```python
from build123d import *
from build123d.topology import SkipClean

# Parameters (mm, degrees)
DODANIE_WYCI_GNI_CIE1_DEPTH = 2
SZKIC_START                 = -28.065385
SZKIC_ZGI_CIA1_DEPTH        = 54
SZKIC_ZGI_CIA1_2_DEPTH      = 15.5
SZKIC_START_2               = 10.434615
SZKIC_ZGI_CIA1_3_DEPTH      = 15.5
SZKIC_START_3               = -56.031828
SZKIC_ZGI_CIA1_4_DEPTH      = 2.423909
SZKIC_START_4               = -12.565385
SZKIC_ZGI_CIA1_5_DEPTH      = 23
SZKIC_ZGI_CIA1_6_DEPTH      = 23
SZKIC_ZGI_CIA2_DEPTH        = 54
SZKIC_ZGI_CIA2_2_DEPTH      = 54
SZKIC_START_5               = 49.968172
SZKIC_ZGI_CIA2_3_DEPTH      = 2
SZKIC9_W                    = 87
SZKIC9_H                    = 28
SZKIC9_W_2                  = 15
SZKIC9_H_2                  = 7
WYTNIJ_WYCI_GNI_CIE1_DEPTH  = 66.825561
SZKIC10_R                   = 1.5
WYTNIJ_WYCI_GNI_CIE2_DEPTH  = 114.762973
ZAOKR_GLENIE2_R             = 1
ZAOKR_GLENIE3_R             = 1


with BuildPart() as part:
    # Szkic1 → Dodanie-wyciągnięcie1 (new body)
    with BuildSketch(Plane.XY):
        with BuildLine():
            Line((-75.531828, 25.934615), (71.468172, 25.934615))
            Line((71.468172, 25.934615), (71.468172, 10.434615))
            ThreePointArc((71.468172, 10.434615), (59.968172, -1.065385), (71.468172, -12.565385))
            Line((71.468172, -12.565385), (71.468172, -28.065385))
            Line((71.468172, -28.065385), (-75.531828, -28.065385))
            Line((-75.531828, -28.065385), (-75.531828, -12.565385))
            ThreePointArc((-75.531828, -12.565385), (-64.031828, -1.065385), (-75.531828, 10.434615))
            Line((-75.531828, 10.434615), (-75.531828, 25.934615))
        make_face()
    extrude(amount=DODANIE_WYCI_GNI_CIE1_DEPTH)

    # Szkic zgięcia1: read off the stored shape, not the designer's step
    # Szkic zgięcia1 outline → Szkic zgięcia1 (cut)
    with BuildSketch(Plane(origin=(0, 0, 0), x_dir=(1, 0, 0), z_dir=(0, 1, 0)).offset(SZKIC_START)):
        with BuildLine():
            Line((-75.531828, -2), (-55.981318, -2))
            ThreePointArc((-55.981318, -2), (-55.112967, -0.563508), (-53.531828, 0))
            Line((-53.531828, 0), (-75.531828, 0))
            Line((-75.531828, 0), (-75.531828, -2))
        make_face()
    extrude(amount=SZKIC_ZGI_CIA1_DEPTH, mode=Mode.SUBTRACT)

    # Szkic zgi_cia1 2 outline → Szkic zgi_cia1 2 (add)
    with BuildSketch(Plane(origin=(0, 0, 0), x_dir=(1, 0, 0), z_dir=(0, 1, 0)).offset(SZKIC_START)):
        with BuildLine():
            ThreePointArc((-55.981318, -2), (-56.019168, -2.248728), (-56.031828, -2.5))
            Line((-56.031828, -2.5), (-56.031828, -22.143806))
            Line((-56.031828, -22.143806), (-54.031828, -22.143806))
            Line((-54.031828, -22.143806), (-54.031828, -2.5))
            ThreePointArc((-54.031828, -2.5), (-53.885381, -2.146447), (-53.531828, -2))
            Line((-53.531828, -2), (-55.981318, -2))
        make_face()
    extrude(amount=SZKIC_ZGI_CIA1_2_DEPTH)

    # Szkic zgi_cia1 3 outline → Szkic zgi_cia1 3 (add)
    with BuildSketch(Plane(origin=(0, 0, 0), x_dir=(1, 0, 0), z_dir=(0, 1, 0)).offset(SZKIC_START_2)):
        with BuildLine():
            ThreePointArc((-55.981318, -2), (-56.019168, -2.248728), (-56.031828, -2.5))
            Line((-56.031828, -2.5), (-56.031828, -22.143806))
            Line((-56.031828, -22.143806), (-54.031828, -22.143806))
            Line((-54.031828, -22.143806), (-54.031828, -2.5))
            ThreePointArc((-54.031828, -2.5), (-53.885381, -2.146447), (-53.531828, -2))
            Line((-53.531828, -2), (-55.981318, -2))
        make_face()
    extrude(amount=SZKIC_ZGI_CIA1_3_DEPTH)

    # Szkic zgi_cia1 4 outline → Szkic zgi_cia1 4 (add)
    with BuildSketch(Plane.YZ.offset(SZKIC_START_3)):
        with BuildLine():
            Line((10.434615, 2), (10.434615, 22.143806))
            ThreePointArc((10.434615, 22.143806), (-1.065385, 10.643806), (-12.565385, 22.143806))
            Line((-12.565385, 22.143806), (-12.565385, 2))
            Line((-12.565385, 2), (10.434615, 2))
        make_face()
    extrude(amount=SZKIC_ZGI_CIA1_4_DEPTH)

    # Szkic zgi_cia1 5 outline → Szkic zgi_cia1 5 (cut)
    with SkipClean():  # the faces are left unmerged after this step: merging them gives an invalid solid
        with BuildSketch(Plane(origin=(0, 0, 0), x_dir=(1, 0, 0), z_dir=(0, 1, 0)).offset(SZKIC_START_4)):
            with BuildLine():
                ThreePointArc((-53.607919, -2.005824), (-53.911331, -2.174459), (-54.031828, -2.5))
                Line((-54.031828, -2.5), (-54.031828, -24))
                Line((-54.031828, -24), (-53.607919, -24))
                Line((-53.607919, -24), (-53.607919, -2.005824))
            make_face()
            with BuildLine():
                Line((-58, -24), (-56.031828, -24))
                Line((-56.031828, -24), (-56.031828, -2.5))
                ThreePointArc((-56.031828, -2.5), (-56.019168, -2.248728), (-55.981318, -2))
                Line((-55.981318, -2), (-58, -2))
                Line((-58, -2), (-58, -24))
            make_face()
        extrude(amount=SZKIC_ZGI_CIA1_5_DEPTH, mode=Mode.SUBTRACT)

    # Szkic zgi_cia1 6 outline → Szkic zgi_cia1 6 (add)
    with SkipClean():  # the faces are left unmerged after this step: merging them gives an invalid solid
        with BuildSketch(Plane(origin=(0, 0, 0), x_dir=(1, 0, 0), z_dir=(0, 1, 0)).offset(SZKIC_START_4)):
            with BuildLine():
                Line((-53.607919, -2), (-53.607919, -2.005824))
                ThreePointArc((-53.607919, -2.005824), (-53.569985, -2.001458), (-53.531828, -2))
                Line((-53.531828, -2), (-53.607919, -2))
            make_face()
        extrude(amount=SZKIC_ZGI_CIA1_6_DEPTH)

    # Szkic zgięcia2: read off the stored shape, not the designer's step
    # Szkic zgięcia2 outline → Szkic zgięcia2 (cut)
    with SkipClean():  # the faces are left unmerged after this step: merging them gives an invalid solid
        with BuildSketch(Plane(origin=(0, 0, 0), x_dir=(1, 0, 0), z_dir=(0, 1, 0)).offset(SZKIC_START)):
            with BuildLine():
                ThreePointArc((49.468172, 0), (51.049311, -0.563508), (51.917662, -2))
                Line((51.917662, -2), (71.468172, -2))
                Line((71.468172, -2), (71.468172, 0))
                Line((71.468172, 0), (49.468172, 0))
            make_face()
        extrude(amount=SZKIC_ZGI_CIA2_DEPTH, mode=Mode.SUBTRACT)

    # Szkic zgi_cia2 2 outline → Szkic zgi_cia2 2 (add)
    with SkipClean():  # the faces are left unmerged after this step: merging them gives an invalid solid
        with BuildSketch(Plane(origin=(0, 0, 0), x_dir=(1, 0, 0), z_dir=(0, 1, 0)).offset(SZKIC_START)):
            with BuildLine():
                Line((49.968172, -22.143806), (51.968172, -22.143806))
                Line((51.968172, -22.143806), (51.968172, -2.5))
                ThreePointArc((51.968172, -2.5), (51.955512, -2.248728), (51.917662, -2))
                Line((51.917662, -2), (49.468172, -2))
                ThreePointArc((49.468172, -2), (49.821725, -2.146447), (49.968172, -2.5))
                Line((49.968172, -2.5), (49.968172, -22.143806))
            make_face()
        extrude(amount=SZKIC_ZGI_CIA2_2_DEPTH)

    # Szkic zgi_cia2 3 outline → Szkic zgi_cia2 3 (cut)
    with SkipClean():  # the faces are left unmerged after this step: merging them gives an invalid solid
        with BuildSketch(Plane.YZ.offset(SZKIC_START_5)):
            with BuildLine():
                Line((10.434615, 22.143806), (-12.565385, 22.143806))
                ThreePointArc((-12.565385, 22.143806), (-1.065385, 10.643806), (10.434615, 22.143806))
            make_face()
        extrude(amount=SZKIC_ZGI_CIA2_3_DEPTH, mode=Mode.SUBTRACT)

    # Szkic9 → Wytnij-wyciągnięcie1 (cut, through all)
    with SkipClean():  # the faces are left unmerged after this step: merging them gives an invalid solid
        with BuildSketch(Plane.XY.offset(2)):
            with Locations((-2.031828, -1.065385)):
                Rectangle(SZKIC9_W, SZKIC9_H)
            with Locations((35.468172, 22.434615)):
                Rectangle(SZKIC9_W_2, SZKIC9_H_2)
            with BuildLine():
                Line((-11.015655, 18.934615), (3.951999, 18.934615))
                ThreePointArc((3.951999, 18.934615), (4.951999, 17.934615), (3.951999, 16.934615))
                Line((3.951999, 16.934615), (-11.015655, 16.934615))
                ThreePointArc((-11.015655, 16.934615), (-12.015655, 17.934615), (-11.015655, 18.934615))
            make_face()
            with BuildLine():
                Line((-9.515655, -19.065385), (5.451999, -19.065385))
                ThreePointArc((5.451999, -19.065385), (6.451999, -20.065385), (5.451999, -21.065385))
                Line((5.451999, -21.065385), (-9.515655, -21.065385))
                ThreePointArc((-9.515655, -21.065385), (-10.515655, -20.065385), (-9.515655, -19.065385))
            make_face()
        extrude(amount=-WYTNIJ_WYCI_GNI_CIE1_DEPTH, mode=Mode.SUBTRACT)

    # Szkic10 → Wytnij-wyciągnięcie2 (cut, through all)
    with SkipClean():  # the faces are left unmerged after this step: merging them gives an invalid solid
        with BuildSketch(Plane.ZY.offset(56.031828)):
            with Locations((7.643806, 14.434615)):
                Circle(SZKIC10_R)
            with Locations((7.643806, -16.565385)):
                Circle(SZKIC10_R)
        extrude(amount=-WYTNIJ_WYCI_GNI_CIE2_DEPTH, mode=Mode.SUBTRACT)

    # Zaokrąglenie2
    zaokr_glenie2_edges = [part.edges().sort_by_distance(p)[0] for p in [
        (27.968172, 25.934615, 1),
        (42.968172, 25.934615, 1),
    ]]
    fillet(zaokr_glenie2_edges, radius=ZAOKR_GLENIE2_R)

    # Zaokrąglenie3
    zaokr_glenie3_edges = [part.edges().sort_by_distance(p)[0] for p in [
        (-45.531828, -15.065385, 1),
        (-45.531828, 12.934615, 1),
        (41.468172, 12.934615, 1),
        (41.468172, -15.065385, 1),
    ]]
    fillet(zaokr_glenie3_edges, radius=ZAOKR_GLENIE3_R)


solid = part.part
```
Geometry: final body of the model. Coordinates: model frame, mm. A direction names the side the tool comes from. Round coordinates to 2 decimals unless told otherwise and drop trailing zeros. Order: outer loops, then holes, each group sorted by start corner. A loop starts at its lowest first (then second) coordinate and runs counter-clockwise, first axis right, second up. Notation, with made-up numbers: M -21.75,15.25 L -12.75,15.25 A25 cw -12.75,52.25 Z; hole C 17,72 d8. An arc over 180 degrees is marked long. Use one line per item in the form item = value. Start each with the question number.
Q1. Cut plane B-B (z = 4.25). Return loops of the section in (x, y).
Q2. Pin query (flat end, axial travel): pin 1 Ø2 at (x, z) = (36.5, 0.5) entering from +Y; pin 2 Ø2 at (y, z) = (0.5, 1) entering from -X; pin 3 Ø2 at (y, z) = (21.5, 0.5) entering from +X. Return the tip coordinate at first contact, or that it passes through.
Q3. Cut plane A-A (y = 22.5). Return loops of the section in (x, z), and give its area (3 significant figures).
Q4. Material intervals for line 1 (X direction, y = 20, z = 16.75); line 2 (Z direction, x = -11, y = 21.5), sorted ascending. Write a range as [from, to].
Q5. Cut plane C-C (x = 7.5). Return loops of the section in (y, z).
Q6. Mould query, pull axis Z, two halves, no side actions, for faces 1 (the face through (-4, 18.935, 1)), 2 (the face through (-55, -20, 22.144)), 3 (the face through (-55.046, 15.922, 7.449)). Classes: +Z half, -Z half, draft (parallel to the pull), parting line (faces both ways), or undercut.
Q7. Cut plane D-D (z = 15.75). Return loops of the section in (x, y).
Q8. Access query for faces 4 (the face through (-1.3, -18.7, 2)), 5 (the face through (-55.13, -1.44, 0.58)), 6 (the face through (-3, -15.065, 1)). Directions: +Z, -Z, +X, -X, +Y, -Y. A direction counts if a zero-diameter tool reaches every point of the face in a straight line with its end or side. Return the directions, or none.
Geometry results:
q1.outline = M -56.03,-28.07 L -54.03,-28.07 L -54.03,25.93 L -56.03,25.93 Z; M 49.97,-28.07 L 51.97,-28.07 L 51.97,25.93 L 49.97,25.93 Z
q2.pin_1 = 18.93
q2.pin_2 = -55.98
q2.pin_3 = 51.76
q3.outline = M -56.03,2.5 A2.5 ccw -55.98,2 A2.5 ccw -53.53,0 L 27.97,0 L 27.97,2 L -53.53,2 A0.5 cw -54.03,2.5 L -54.03,22.14 L -56.03,22.14 Z; M 42.97,0 L 49.47,0 A2.5 ccw 51.92,2 A2.5 ccw 51.97,2.5 L 51.97,22.14 L 49.97,22.14 L 49.97,2.5 A0.5 cw 49.47,2 L 42.97,2 Z
q3.area = 264 mm^2
q4.line_1 = [-56.03, -54.03], [49.97, 51.97]
q4.line_2 = [0, 2]
q5.outline = M -28.07,0 L -15.07,0 L -15.07,2 L -28.07,2 Z; M 12.93,0 L 25.93,0 L 25.93,2 L 12.93,2 Z
q6.face_1 = draft
q6.face_2 = +Z half
q6.face_3 = undercut
q7.outline = M -56.03,-28.07 L -54.03,-28.07 L -54.03,-10.62 L -56.03,-10.62 Z; M -56.03,8.49 L -54.03,8.49 L -54.03,25.93 L -56.03,25.93 Z; M 49.97,-28.07 L 51.97,-28.07 L 51.97,-10.62 L 49.97,-10.62 Z; M 49.97,8.49 L 51.97,8.49 L 51.97,25.93 L 49.97,25.93 Z
q8.face_4 = +Z, +Y, -Y
q8.face_5 = -Z, -X, +Y, -Y
q8.face_6 = +Z, -Z
